Input: part model. Units: mm. Frame: model coordinates. Face numbers are marked on the shaded views. Give positions to 0.01 mm unless a question says otherwise; leave off trailing zeros. Order: outer loops, then holes, each group sorted by start corner. A loop starts at its lowest first (then second) coordinate and runs counter-clockwise, first axis right, second up. Notation, with made-up numbers: M 8,28 L 58,28 A28 cw 58,59 Z; hole C 1.5,-18 d9. An arc over 180 degrees is marked long. Use a Markdown table: item, result.
from build123d import *

# Parameters (mm, degrees)
BOSS_EXTRUDE1_DEPTH = 229
SKETCH3_R           = 44.45
CUT_EXTRUDE1_DEPTH  = 78
SKETCH4_R           = 28.575
CUT_EXTRUDE2_DEPTH  = 238.531050602


with BuildPart() as part:
    # Sketch2 → Boss-Extrude1 (new body)
    with BuildSketch(Plane.XY):
        with BuildLine():
            Line((0, 0), (0, 164))
            ThreePointArc((0, 164), (-57.982756057, 139.982756057), (-82, 82))
            Line((-82, 82), (-82, 39.837168574))
            Line((-82, 39.837168574), (-13, 0))
            Line((-13, 0), (0, 0))
        make_face()
    extrude(amount=BOSS_EXTRUDE1_DEPTH)

    # Sketch3 → Cut-Extrude1 (cut)
    with BuildSketch(Plane.XY.offset(229)):
        with Locations((0, 82)):
            Circle(SKETCH3_R)
    extrude(amount=-CUT_EXTRUDE1_DEPTH, mode=Mode.SUBTRACT)

    # Sketch4 → Cut-Extrude2 (cut, through all)
    with BuildSketch(Plane.XY.offset(151)):
        with Locations((0, 82)):
            Circle(SKETCH4_R)
    extrude(amount=-CUT_EXTRUDE2_DEPTH, mode=Mode.SUBTRACT)


solid = part.part
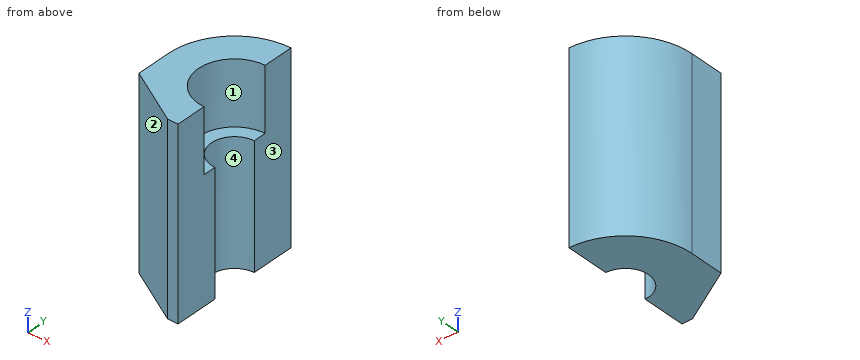
1) Cut plane A-A on z = 174. Return loops of the section in (x, y), and give its area (3 significant figures).
Response values:
| item | result |
|---|---|
| outline | M -82,39.84 L -13,0 L 0,0 L 0,37.55 A44.45 cw 0,126.45 L 0,164 A82 ccw -82,82 Z |
| area | 7,530 mm² |
2) Material intervals for line 1 (Z direction, x = -35, y = 58); line 2 (Y direction, x = -25, z = 48.5); line 3 (Y direction, x = -23.5, z = 136), sorted ascending. Write a range as from..to.
Response values:
| item | result |
|---|---|
| line 1 | z = 0..151 |
| line 2 | y = 6.93..68.16, 95.84..160.1 |
| line 3 | y = 6.06..65.74, 98.26..160.56 |
3) Cut plane B-B on x = -8.5. Return loops of the section in (y, z), and give its area (3 significant figures).
Response values:
| item | result |
|---|---|
| outline | M 0,0 L 54.72,0 L 54.72,151 L 38.37,151 L 38.37,229 L 0,229 Z; M 109.28,0 L 163.56,0 L 163.56,229 L 125.63,229 L 125.63,151 L 109.28,151 Z |
| area | 22,400 mm² |
4) Mould query, pull axis Y, two halves, no side actions, for the marked faces 1, 2, 3 and 4. Classes: released by +Y, released by -Y, zero draft, split by the parting line, or undercut.
Response values:
| item | result |
|---|---|
| face 1 | undercut |
| face 2 | released by -Y |
| face 3 | zero draft |
| face 4 | undercut |
5) Cut plane D-D on y = 103. Return loops of the section in (x, z), and give its area (3 significant figures).
Response values:
| item | result |
|---|---|
| outline | M -79.27,0 L -19.38,0 L -19.38,151 L -39.18,151 L -39.18,229 L -79.27,229 Z |
| area | 12,200 mm² |
6) First-contact query: pin 1 Ø5 at (x, z) = (-25.5, 202) entering from +Y; pin 2 Ø3 at (y, z) = (85.5, 138) entering from +X; pin 3 Ø3 at (x, z) = (-30.5, 120) entering from -Y. Flat tips, straight axial feed; report the tip coordinate or a pass-through.
Response values:
| item | result |
|---|---|
| pin 1 | stops at y = 160.71 |
| pin 2 | stops at x = -28.13 |
| pin 3 | stops at y = 9.24 |
7) Cut plane C-C on z = 41.5. Return loops of the section in (x, y) (3 decimals).
Response values:
| item | result |
|---|---|
| outline | M -82,39.837 L -13,0 L 0,0 L 0,53.425 A28.575 cw 0,110.575 L 0,164 A82 ccw -82,82 Z |
